Geometry: final body of the model. Coordinates: model frame, mm. A direction names the side the tool comes from. Give positions to 0.01 mm unless a question says otherwise; leave off trailing zeros. Loops run counter-clockwise (first coordinate to the right, second up) from the corner with the lowest first, then second, coordinate; pieces in that order, holes last. Notation, with made-up numbers: (21, 68.25) - (68, 68.25) arc R21 cw to (68, 72.25) - close; hole circle Ø3 at (-5, 10). An arc over 180 degrees is marked (long way). Use one line per item in the form item = value.
```python
from build123d import *

# Parameters (mm, degrees)
BOSS_EXTRUDE1_DEPTH = 1.524


with BuildPart() as part:
    # Sketch1 → Boss-Extrude1 (new body)
    with BuildSketch(Plane.XY):
        with BuildLine():
            Line((1.524, 62.176210227), (1.524, 64.48445576))
            Line((1.524, 64.48445576), (3.048, 64.48445576))
            Line((3.048, 64.48445576), (3.048, 66.00845576))
            Line((3.048, 66.00845576), (4.572, 66.00845576))
            Line((4.572, 66.00845576), (4.572, 64.48445576))
            Line((4.572, 64.48445576), (6.898856883, 64.48445576))
            ThreePointArc((6.898856883, 64.48445576), (7.354991053, 64.200075123), (7.300433388, 63.665328277))
            Line((7.300433388, 63.665328277), (1.524, 56.209606557))
            Line((1.524, 56.209606557), (0, 56.209606557))
            Line((0, 56.209606557), (-5.776433388, 63.665328277))
            ThreePointArc((-5.776433388, 63.665328277), (-5.830991053, 64.200075123), (-5.374856883, 64.48445576))
            Line((-5.374856883, 64.48445576), (-3.048, 64.48445576))
            Line((-3.048, 64.48445576), (-3.048, 66.00845576))
            Line((-3.048, 66.00845576), (-1.524, 66.00845576))
            Line((-1.524, 66.00845576), (-1.524, 64.48445576))
            Line((-1.524, 64.48445576), (0, 64.48445576))
            Line((0, 64.48445576), (0, 62.176210227))
            Line((0, 62.176210227), (1.524, 62.176210227))
        make_face()
    extrude(amount=BOSS_EXTRUDE1_DEPTH)


solid = part.part
```
(1) Access query for faces 4 (the face through (-2.85, 59.89, 0.75)), 5 (the face through (-1.524, 65, 1)), 6 (the face through (4, 66.008, 1)), 7 (the face through (-4, 64.484, 1)), 8 (the face through (4.572, 65, 1)). Directions: +Z, -Z, +X, -X, +Y, -Y. A direction counts if a zero-diameter tool reaches every point of the face in a straight line with its end or side. Return the directions, or none.
Solution:
face_4 = +Z, -Z, -X, -Y
face_5 = +Z, -Z, +Y
face_6 = +Z, -Z, +X, -X, +Y
face_7 = +Z, -Z, -X, +Y
face_8 = +Z, -Z, +X, +Y
(2) Cut plane C-C (x = -4.25). Return the cut outline in (y, z).
Solution:
outline = (61.7, 0) - (64.48, 0) - (64.48, 1.52) - (61.7, 1.52) - close
(3) Cut plane D-D (y = 57.25). Return the cut outline in (x, z), plus the area to 3 significant figures.
Solution:
outline = (-0.81, 0) - (2.33, 0) - (2.33, 1.52) - (-0.81, 1.52) - close
area = 4.78 mm2
(4) Pull-direction query (X, two-part tool) for faces 1 (the face through (1.524, 63, 1)), 2 (the face through (1, 56.21, 1)), 3 (the face through (-5.834, 64.193, 0.751)); classes: released by +X, released by -X, zero draft, split by the parting line, or undercut.
Solution:
face_1 = undercut
face_2 = zero draft
face_3 = released by -X
(5) Pin query (flat end, axial travel): P1, Ø0.5, axis at x = -5, z = 1, coming from the +Y side; P2, Ø0.8, axis at y = 63, z = 0.5, coming from the +X side; P3, Ø0.8, axis at y = 65, z = 0.5, coming from the -X side. Return the tip coordinate at first contact, or that it passes through.
Solution:
P1 = 64.48
P2 = 7.09
P3 = -3.05
(6) Cut plane B-B (y = 64). Return the cut outline in (x, z), plus the area to 3 significant figures.
Solution:
outline = (-5.88, 0) - (0, 0) - (0, 1.52) - (-5.88, 1.52) - close; (1.52, 0) - (7.41, 0) - (7.41, 1.52) - (1.52, 1.52) - close
area = 17.9 mm2
(7) Material intervals for L1, parallel to X at y = 63.5, z = 0.85; L2, parallel to X at y = 59, z = 0.95; L3, parallel to Y at x = 2.75, z = 0.7, sorted ascending. Write a range as from..to.
Solution:
L1 = -5.65..0, 1.52..7.17
L2 = -2.16..3.69
L3 = 57.79..64.48
(8) Cut plane A-A (z = 0.4). Return the cut outline in (x, y), plus the area to 3 significant figures.
Solution:
outline = (-5.78, 63.67) - (0, 56.21) - (1.52, 56.21) - (7.3, 63.67) arc R0.51 ccw to (6.9, 64.48) - (4.57, 64.48) - (4.57, 66.01) - (3.05, 66.01) - (3.05, 64.48) - (1.52, 64.48) - (1.52, 62.18) - (0, 62.18) - (0, 64.48) - (-1.52, 64.48) - (-1.52, 66.01) - (-3.05, 66.01) - (-3.05, 64.48) - (-5.37, 64.48) arc R0.51 ccw to start
area = 66.3 mm2
